Design review of the part built by this model. Coordinates are the model's own, in mm. Face numbers are marked on the shaded views. A direction names the side the tool comes from. Coordinates: 2 decimals unless noted, no trailing zeros. Order: outer loops, then holes, each group sorted by start corner. A loop starts at its lowest first (then second) coordinate and runs counter-clockwise, first axis right, second up. Notation, with made-up numbers: M 44.25,25 L 68.25,25 A31 ccw 68.25,60 Z; hole C 38.5,80.25 d11. An arc over 180 degrees is marked long. Answer in a Markdown table with one row per item.
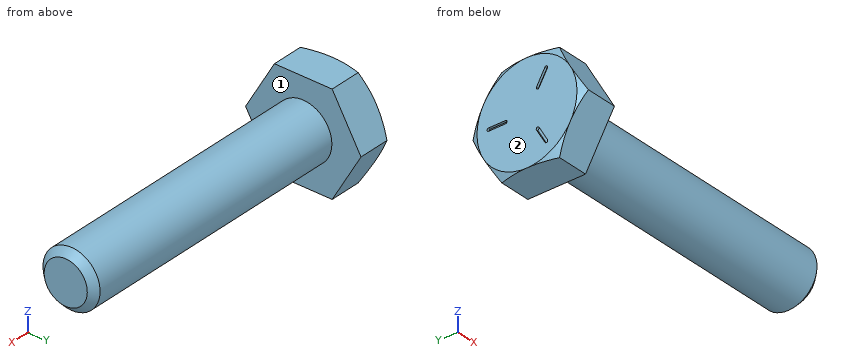
from build123d import *

# Parameters (mm, degrees)
SKETCH5_R           = 3.175
BOSS_EXTRUDE3_DEPTH = 31.75
CHAMFER1_SIZE       = 0.77724
BOSS_EXTRUDE4_DEPTH = 3.96875
SKETCH8_OUTSIDE_W   = 148.218
SKETCH8_OUTSIDE_H   = 149.938
SKETCH8_OUTSIDE_R   = 5.55625
CUT_EXTRUDE3_DEPTH  = 36.71875
CUT_EXTRUDE3_TAPER  = 60
CUT_EXTRUDE4_DEPTH  = 0.254
CIRPATTERN1_COUNT   = 3


with BuildPart() as part:
    # Sketch5 → Boss-Extrude3 (new body)
    with BuildSketch(Plane(origin=(17.859375, 0, 0), x_dir=(0, 0, -1), z_dir=(1, 0, 0))):
        Circle(SKETCH5_R)
    extrude(amount=-BOSS_EXTRUDE3_DEPTH)

    # Chamfer1
    chamfer1_edges = [part.edges().sort_by_distance(p)[0] for p in [
        (17.859375, 0, 3.175),
    ]]
    chamfer(chamfer1_edges, length=CHAMFER1_SIZE)

    # Sketch6 → Boss-Extrude4 (add)
    with BuildSketch(Plane.ZY.offset(13.890625)):
        Polygon((5.55625, 3.207902433), (0, 6.415804866), (-5.55625, 3.207902433), (-5.55625, -3.207902433), (0, -6.415804866), (5.55625, -3.207902433), align=None)
    extrude(amount=BOSS_EXTRUDE4_DEPTH)

    # Sketch8 outside → Cut-Extrude3 (cut, through all)
    with BuildSketch(Plane.ZY.offset(17.859375)):
        Rectangle(SKETCH8_OUTSIDE_W, SKETCH8_OUTSIDE_H)
        Circle(SKETCH8_OUTSIDE_R, mode=Mode.SUBTRACT)
    extrude(amount=-CUT_EXTRUDE3_DEPTH, taper=CUT_EXTRUDE3_TAPER, mode=Mode.SUBTRACT)

    # Sketch12 → Cut-Extrude4 (cut)
    with BuildSketch(Plane.ZY.offset(17.859375)):
        with BuildLine():
            Line((0.1666875, 4.2783125), (0.1666875, 2.3891875))
            ThreePointArc((0.1666875, 2.3891875), (0, 2.2225), (-0.1666875, 2.3891875))
            Line((-0.1666875, 2.3891875), (-0.1666875, 4.2783125))
            ThreePointArc((-0.1666875, 4.2783125), (0, 4.445), (0.1666875, 4.2783125))
        make_face()
    cut_extrude4 = extrude(amount=-CUT_EXTRUDE4_DEPTH, mode=Mode.SUBTRACT)

    # CirPattern1: Cut-Extrude4 ×3 about axis
    cirpattern1_axis = Axis((0, 0, 0), (1, 0, 0))
    for i in range(1, CIRPATTERN1_COUNT):
        add(cut_extrude4.rotate(cirpattern1_axis, i * 360 / CIRPATTERN1_COUNT), mode=Mode.SUBTRACT)


solid = part.part
(1) Insertion check: pin 1 Ø3 at (x, z) = (9.5, -1.5) entering from -Y (3 decimals); pin 2 Ø1 at (x, z) = (-4.5, 0.5) entering from +Y (3 decimals); pin 3 Ø6 at (x, y) = (10, 0) entering from +Z (3 decimals); pin 4 Ø2 at (y, z) = (3, 0) entering from -X. Each pin has a flat end and moves straight along its axis. Give the tip position at first contact, or say it passes through.
Return value:
| item | result |
|---|---|
| pin 1 | stops at y = -3.175 |
| pin 2 | stops at y = 3.175 |
| pin 3 | stops at z = 3.175 |
| pin 4 | stops at x = -17.86 |
(2) For the marked faces 1 and 2, list the 3-axis set-ups (+Z, -Z, +X, -X, +Y, -Y) from which the entire face can be reached by the end or side of a thin tool; tool diameter is ignored.
Return value:
| item | result |
|---|---|
| face 1 | +X |
| face 2 | +Z, -Z, -X, +Y, -Y |
(3) Add section A-A, the plane x = 5. Give the boundary of the cut face in (y, z) (3 decimals), and give its area (3 significant figures).
Return value:
| item | result |
|---|---|
| outline | C 0,0 d6.35 |
| area | 31.7 mm2 |
(4) For line 1 along X through (y, z) = (0, 4); line 2 along Y through (x, z) = (-15.5, 0.5); line 3 along Y through (x, z) = (-9, 2.5), list the stretches that pass through material, from the lowest coordinate up. Write a range as from..to.
Return value:
| item | result |
|---|---|
| line 1 | x = -17.86..-13.89 |
| line 2 | y = -6.13..6.13 |
| line 3 | y = -1.96..1.96 |
